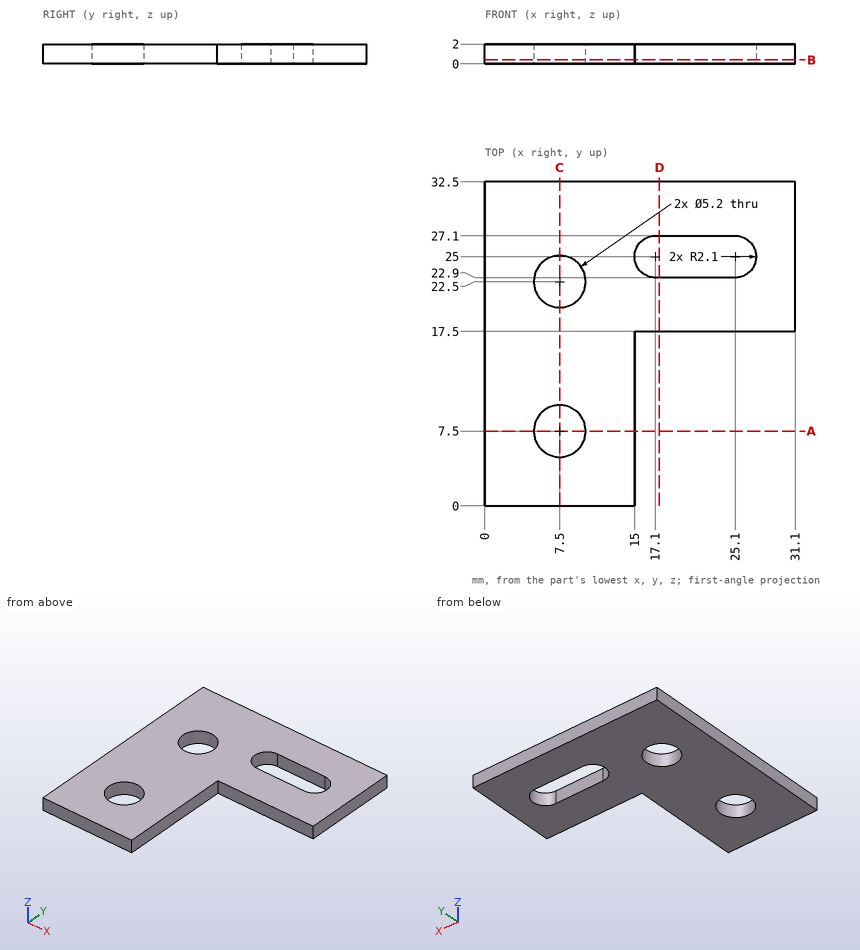
Study the drawing (mm; zero at the part's minimum x, y, z) and answer. Coordinates: 2 decimals unless noted, no trailing zeros. Write each loop counter-clockwise with the first axis right and the second up, starting at its lowest first coordinate (ties: lowest second). Pieces come first, ordered by that corner, then holes. Notation, with made-up numbers: (23.5, -9.75) - (53.5, -9.75) arc R13 ccw to (53.5, -4.75) - close; hole circle Ø7 at (77.25, -22.75). An arc over 180 degrees is marked (long way). Put each result on its own line as item: value.
1. A flat-ended cylindrical pin translates along its axis: pin 1 Ø6 at (x, y) = (7.5, 7.5) entering from +Z. Find the tip coordinate at first contact, or state that the pin passes through.
Answer sheet:
pin 1: stops at z = 2
2. Find the intervals of material crossed by line 1 along Y through (x, z) = (7.5, 1.6); line 2 along Y through (x, z) = (22, 1.1); line 3 along X through (y, z) = (23.5, 0.2), in increasing order. Write a range as from..to.
Answer sheet:
line 1: y = 0..4.9, 10.1..19.9, 25.1..32.5
line 2: y = 17.5..22.9, 27.1..32.5
line 3: x = 0..5.1, 9.9..15.63, 26.57..31.1
3. The part is cut by section D-D on x = 17.5. Give the vertices of the cut face in (y, z).
Answer sheet:
outline: (17.5, 0) - (22.9, 0) - (22.9, 2) - (17.5, 2) - close; (27.1, 0) - (32.5, 0) - (32.5, 2) - (27.1, 2) - close
4. The part is cut by section B-B on z = 0.4. Give the vertices of the cut face in (x, y), plus the area to 3 significant figures.
Answer sheet:
outline: (0, 0) - (15, 0) - (15, 17.5) - (31.1, 17.5) - (31.1, 32.5) - (0, 32.5) - close; hole circle Ø5.2 at (7.5, 7.5); hole circle Ø5.2 at (7.5, 22.5); hole (17.1, 22.9) - (25.1, 22.9) arc R2.1 ccw to (25.1, 27.1) - (17.1, 27.1) arc R2.1 ccw to start
area: 639 mm^2
5. The part is cut by section C-C on x = 7.5. Give the vertices of the cut face in (y, z).
Answer sheet:
outline: (0, 0) - (4.9, 0) - (4.9, 2) - (0, 2) - close; (10.1, 0) - (19.9, 0) - (19.9, 2) - (10.1, 2) - close; (25.1, 0) - (32.5, 0) - (32.5, 2) - (25.1, 2) - close
6. The part is cut by section A-A on y = 7.5. Give the vertices of the cut face in (x, z), plus the area to 3 significant figures.
Answer sheet:
outline: (0, 0) - (4.9, 0) - (4.9, 2) - (0, 2) - close; (10.1, 0) - (15, 0) - (15, 2) - (10.1, 2) - close
area: 19.6 mm^2
